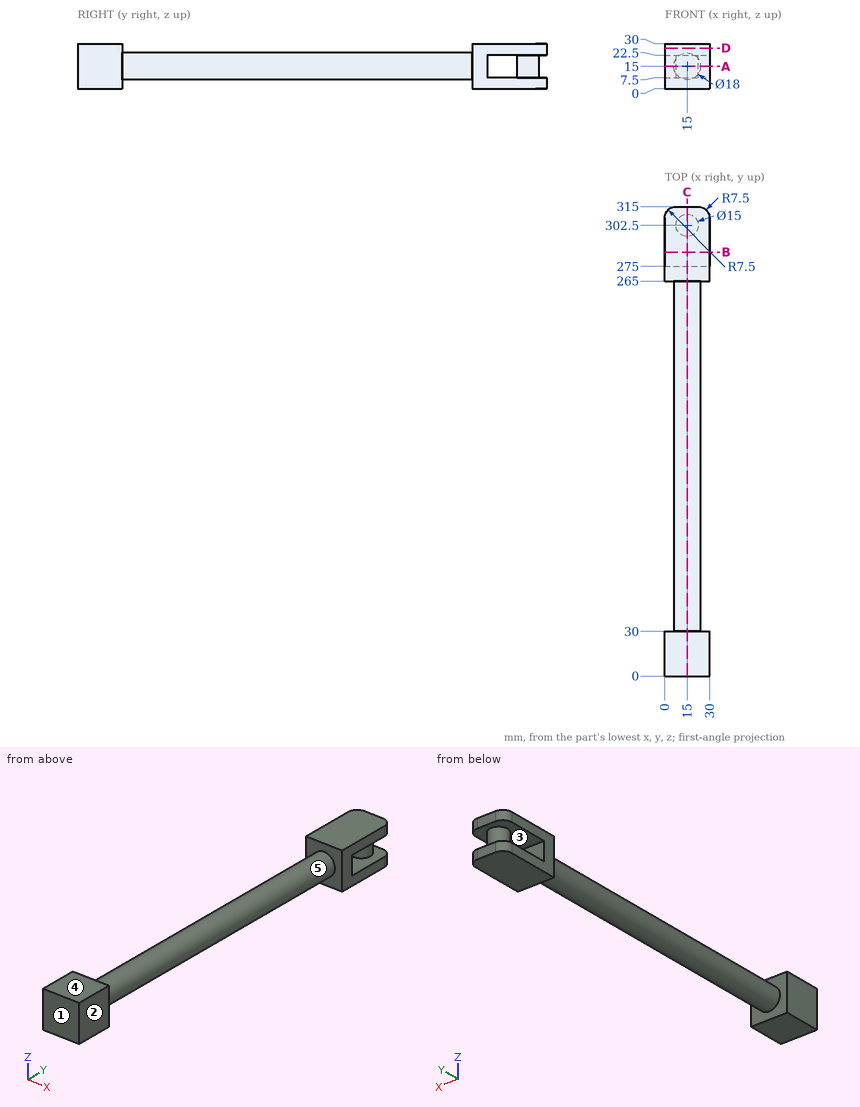
Answer from the drawing. Dimensions are ordinates in mm from the lowest x, y and z of the part. A direction names the side the tool comes from. Give positions to 0.01 mm unless a question says otherwise; leave off trailing zeros. Write each loop counter-clockwise with the first axis right and the second up, starting at its lowest first coordinate (ties: lowest second). Pieces come first, ordered by that corner, then holes.
1) Section A-A (z = 15) is taken. Write down the section's boundary in (x, y), and give its area (3 significant figures).
2) Given P1, Ø1.5, axis at x = 6.5, z = 10.5, coming from the +Y side; P2, Ø12, axis at y = 238, z = 11.5, coming from the +X side; P3, Ø12, axis at x = 16.5, y = 208, coming from the -Z side; P4, Ø5, axis at x = 16.5, z = 14.5, coming from the -Y side, each flat-ended and moving along its own axis, determine where each tip first touches the part or whether it passes through.
3) For a pull along Y with two mould halves and no side action, classify the marked faces 1, 2 and 3 as pulls with the +Y half, pulls with the -Y half, needs draft (parallel to the pull), parting line crosses it, or undercut.
4) A tool of negligible diameter and unlimited length cuts with its end or side. For the marked faces 4 and 5, from which of +Z, -Z, +X, -X, +Y, -Y can it reach the whole face along a straight path? Write none if from no direction.
5) Section B-B (y = 284.5) is taken. Write down the section's boundary in (x, z).
6) Section C-C (x = 15) is taken. Write down the section's boundary in (y, z).
7) Find the intervals of material crossed by L1, parallel to Y at x = 15.5, z = 12.25; L2, parallel to Y at x = 6, z = 18; L3, parallel to Z at x = 8, y = 278.5, in increasing order.
8) Section D-D (z = 27.25) is taken. Write down the section's boundary in (x, y).
Response:
1. outline: (0, 0) - (30, 0) - (30, 30) - (24, 30) - (24, 265) - (30, 265) - (30, 275) - (0, 275) - (0, 265) - (6, 265) - (6, 30) - (0, 30) - close; circle Ø15 at (15, 302.5)
1. area: 5,610 mm2
2. P1: stops at y = 275
2. P2: stops at x = 24
2. P3: stops at z = 6
2. P4: stops at y = 0
3. face 1: pulls with the -Y half
3. face 2: needs draft
3. face 3: undercut
4. face 4: +Z, +X, -X, +Y, -Y
4. face 5: none
5. outline: (0, 0) - (30, 0) - (30, 7.5) - (0, 7.5) - close; (0, 22.5) - (30, 22.5) - (30, 30) - (0, 30) - close
6. outline: (0, 0) - (30, 0) - (30, 6) - (265, 6) - (265, 0) - (315, 0) - (315, 7.5) - (310, 7.5) - (310, 22.5) - (315, 22.5) - (315, 30) - (265, 30) - (265, 24) - (30, 24) - (30, 30) - (0, 30) - close; hole (275, 7.5) - (295, 7.5) - (295, 22.5) - (275, 22.5) - close
7. L1: y = 0 to 275, 295.02 to 309.98
7. L2: y = 0 to 30, 265 to 275
7. L3: z = 0 to 7.5, 22.5 to 30
8. outline: (0, 0) - (30, 0) - (30, 30) - (0, 30) - close; (0, 265) - (30, 265) - (30, 307.5) arc R7.5 ccw to (22.5, 315) - (7.5, 315) arc R7.5 ccw to (0, 307.5) - close
